```python
from build123d import *

# Parameters (mm, degrees)
F1_DEPTH = 100
F2_DEPTH = 15
F2_TAPER = -45


with BuildPart() as f1:
    # F0 (on Front) → F1 (new body)
    with BuildSketch(Plane.XZ):
        Polygon((-0.1822671791, 11.2663906845), (-8.618093033, 2.1458949195), (-0.1375637321, -15.4114313191), (8.9392346026, 1.9508140394), align=None)
    extrude(amount=F1_DEPTH)

    # F1_face (on face) → F2 (join)
    with BuildSketch(Plane(origin=(0.0560458234, 0, -0.7001079654), x_dir=(1, 0, 0), z_dir=(0, 1, 0))):
        Polygon((-8.6741388563, -2.8460028849), (-0.2383130025, -11.9664986499), (8.8831887792, -2.6509220048), (-0.1936095555, 14.7113233537), align=None)
    extrude(amount=F2_DEPTH, taper=F2_TAPER)


solid = f1.part
```
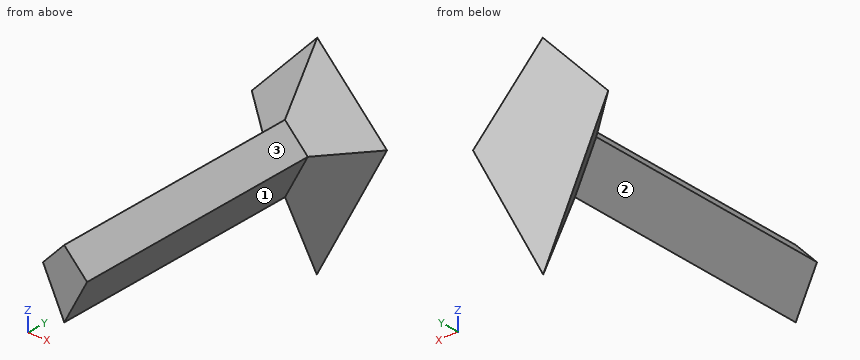
Could you check a few things on this model? Use its own coordinates, in mm. Face numbers are marked on the shaded views. A direction names the side the tool comes from. Round coordinates to 2 decimals unless told otherwise and drop trailing zeros. Loops run counter-clockwise (first coordinate to the right, second up) from the corner with the lowest first, then second, coordinate; pieces in that order, holes last.
Q1. I want a section at A-A (y = -85). Write out the boundary of the cut face in (x, z), and give its area (3 significant figures).
Q2. For P1, Ø1, axis at y = -43.5, z = 8, coming from the +X side; P2, Ø8, axis at x = -5, y = -18, coming from the +Z side; P3, Ø1.5, axis at x = 0, z = -22.5, coming from the -Y side (3 decimals), each with a flat end and sliding along its axis, tell me the tip position at first contact or that it passes through.
Q3. Please list where these lines run through material, in increasing order: L1, parallel to X at y = -57.5, z = 10.5; L2, parallel to Z at x = -2, y = -90; L3, parallel to Y at x = -5.5, z = -35.
Q4. On a 3-axis mill with a long thin cutter (end or side, diameter ignored), from which of +Z, -Z, +X, -X, +Y, -Y can I reach the whole of each face in a straight line? I mean the marked faces 1, 2 and 3. Say none if no direction works.
Answer below:
1. outline: (-8.62, 2.15) - (-0.14, -15.41) - (8.94, 1.95) - (-0.18, 11.27) - close
1. area: 234 mm2
2. P1: stops at x = 3.51
2. P2: stops at z = 10.38
2. P3: stops at y = 2.865
3. L1: x = -0.89 to 0.57
3. L2: z = -11.56 to 9.3
3. L3: y = 13.35 to 15
4. face 1: -Z, +X, -Y
4. face 2: -Z, -X, -Y
4. face 3: +Z, +X, -Y
